Study the drawing (mm; zero at the part's minimum x, y, z) and answer. Coordinates: 2 decimals unless noted, no trailing zeros. Loops run counter-clockwise (first coordinate to the right, second up) from the corner with the lowest first, then second, coordinate; pieces in that order, holes last. Notation, with made-up numbers: (50, -30) -> (78, -30) arc R19 ccw to (78, 5) -> close; hole circle Ø9 at (52.25, -10). An arc over 180 degrees is marked (long way). One line per question, with ' | ' between items.
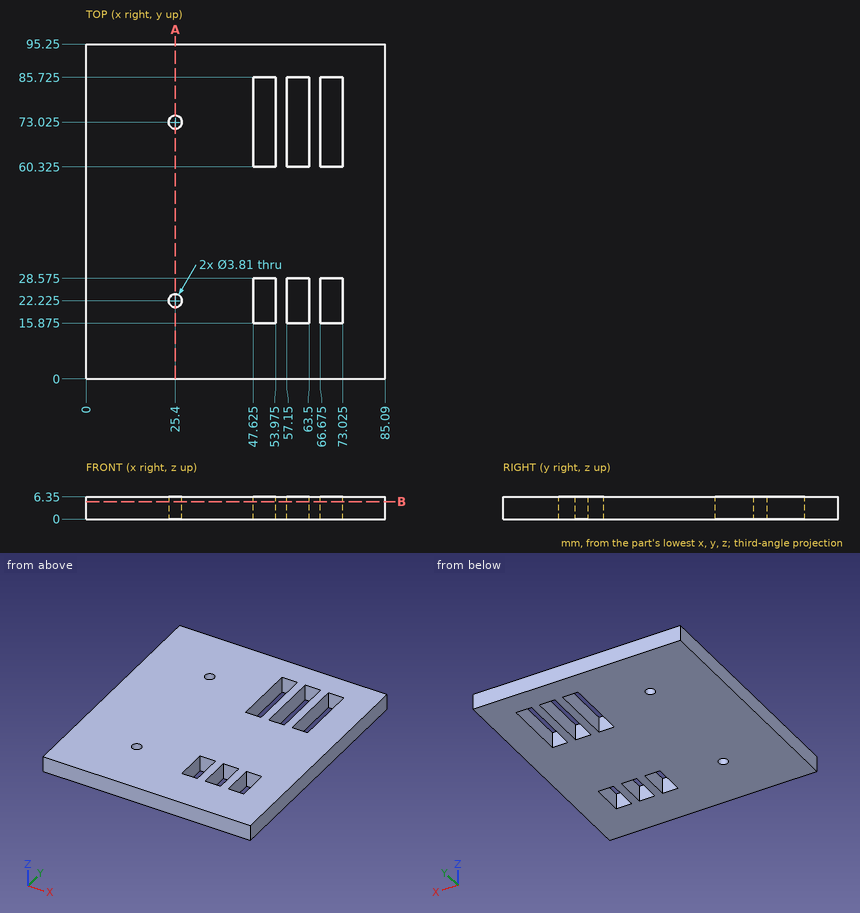
1) Find section B-B (z = 5). State how many separate pieces and enclosed holes the cut face has, plus the area to 3 significant figures.
Check values:
separate pieces: 1 | enclosed holes: 8 | area: 7,360 mm^2
2) Find section A-A (x = 25.4). Write down the section's boundary in (y, z), plus the area to 3 significant figures.
Check values:
outline: (0, 0) -> (20.32, 0) -> (20.32, 6.35) -> (0, 6.35) -> close; (24.13, 0) -> (71.12, 0) -> (71.12, 6.35) -> (24.13, 6.35) -> close; (74.93, 0) -> (95.25, 0) -> (95.25, 6.35) -> (74.93, 6.35) -> close | area: 556 mm^2
3) Flat-ended cylindrical pins translate along their axes: pin 1 (6 mm diameter, centred on x = 25.4, y = 22.225, fed in from +Z); pin 2 (3.5 mm diameter, centred on x = 25.4, y = 73.025, fed in from +Z). Find the tip coordinate at first contact, or state that the pin passes through.
Check values:
pin 1: stops at z = 6.35 | pin 2: passes through
4) Find the intervals of material crossed by line 1 along Y through (x, z) = (25.4, 2.25); line 2 along X through (y, z) = (16, 0.5) (3 decimals); line 3 along X through (y, z) = (23, 4.75) (3 decimals), in increasing order.
Check values:
line 1: y = 0 to 20.32, 24.13 to 71.12, 74.93 to 95.25 | line 2: x = 0 to 47.625, 53.975 to 57.15, 63.5 to 66.675, 73.025 to 85.09 | line 3: x = 0 to 23.66, 27.14 to 47.625, 53.975 to 57.15, 63.5 to 66.675, 73.025 to 85.09
